Geometry: final body of the model. Coordinates: model frame, mm. Round coordinates to 2 decimals unless told otherwise and drop trailing zeros. Loops run counter-clockwise (first coordinate to the right, second up) from the corner with the lowest first, then second, coordinate; pieces in that order, holes last. Notation, with made-up numbers: (27, 67.5) -> (38, 67.5) arc R26 ccw to (38, 86.5) -> close; hole circle Ø10 at (68, 53). An arc over 180 degrees is marked (long way). Answer in a Markdown table with one row per item.
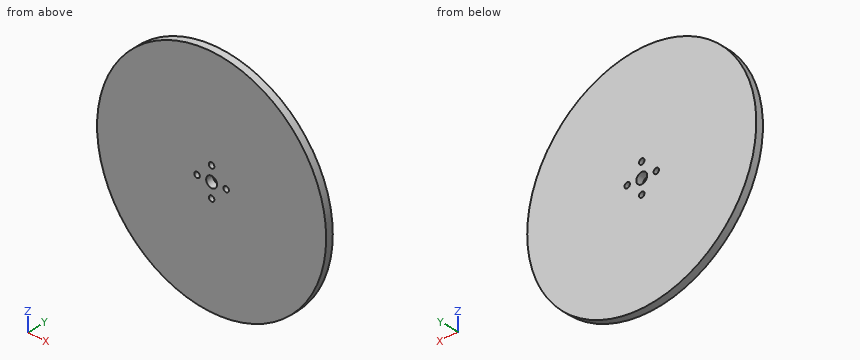
```python
from build123d import *

# Parameters (mm, degrees)
SKETCH_1_R          = 63
EXTRUDE_1_DEPTH     = 4
SKETCH_2_R          = 1.5
SKETCH_2_R_2        = 3
CUT_EXTRUDE_1_DEPTH = 5


with BuildPart() as part:
    # 草图1 → 凸台-拉伸1 (new body)
    with BuildSketch(Plane(origin=(0, 0, 0), x_dir=(1, 0, 0), z_dir=(0, 1, 0))):
        Circle(SKETCH_1_R)
    extrude(amount=EXTRUDE_1_DEPTH)

    # 草图2 → 切除-拉伸1 (cut, through all)
    with BuildSketch(Plane(origin=(0, 4, 0), x_dir=(1, 0, 0), z_dir=(0, 1, 0))):
        with Locations((8, 0)):
            Circle(SKETCH_2_R)
        with Locations((0, 8)):
            Circle(SKETCH_2_R)
        with Locations((-8, 0)):
            Circle(SKETCH_2_R)
        with Locations((0, -8)):
            Circle(SKETCH_2_R)
        Circle(SKETCH_2_R_2)
    extrude(amount=-CUT_EXTRUDE_1_DEPTH, mode=Mode.SUBTRACT)


solid = part.part
```
Item 1: Cut plane A-A (z = 0). Output: boundary loops of the cut face in (x, y), then the cut area to 3 significant figures.
Answer:
| item | result |
|---|---|
| outline | (-63, 0) -> (-9.5, 0) -> (-9.5, 4) -> (-63, 4) -> close; (-6.5, 0) -> (-3, 0) -> (-3, 4) -> (-6.5, 4) -> close; (3, 0) -> (6.5, 0) -> (6.5, 4) -> (3, 4) -> close; (9.5, 0) -> (63, 0) -> (63, 4) -> (9.5, 4) -> close |
| area | 456 mm² |
Item 2: Cut plane C-C (y = 3.25). Output: boundary loops of the cut face in (x, z), then the cut area to 3 significant figures.
Answer:
| item | result |
|---|---|
| outline | circle Ø126 at (0, 0); hole circle Ø3 at (-8, 0); hole circle Ø6 at (0, 0); hole circle Ø3 at (0, -8); hole circle Ø3 at (0, 8); hole circle Ø3 at (8, 0) |
| area | 12,400 mm² |
Item 3: Line query: probe 1 along X at (y, z) = (0.95, 0); probe 2 along X at (y, z) = (3.15, -8). Output: solid intervals per line, ascending. Write a range as [from, to].
Answer:
| item | result |
|---|---|
| probe 1 | x = [-63, -9.5], [-6.5, -3], [3, 6.5], [9.5, 63] |
| probe 2 | x = [-62.49, -1.5], [1.5, 62.49] |
Item 4: Pin query (flat end, axial travel): pin 1 Ø1.5 at (y, z) = (3.5, -20.5) entering from -X; pin 2 Ø2 at (x, y) = (46, 3.5) entering from +Z; pin 3 Ø1 at (x, y) = (49, 2) entering from +Z. Return the tip coordinate at first contact, or that it passes through.
Answer:
| item | result |
|---|---|
| pin 1 | stops at x = -59.82 |
| pin 2 | stops at z = 44.09 |
| pin 3 | stops at z = 40.21 |
Item 5: Cut plane D-D (z = -34.5). Output: boundary loops of the cut face in (x, y).
Answer:
| item | result |
|---|---|
| outline | (-52.71, 0) -> (52.71, 0) -> (52.71, 4) -> (-52.71, 4) -> close |
Item 6: Cut plane B-B (x = -8). Output: boundary loops of the cut face in (y, z), then the cut area to 3 significant figures.
Answer:
| item | result |
|---|---|
| outline | (0, -62.49) -> (4, -62.49) -> (4, -1.5) -> (0, -1.5) -> close; (0, 1.5) -> (4, 1.5) -> (4, 62.49) -> (0, 62.49) -> close |
| area | 488 mm² |
